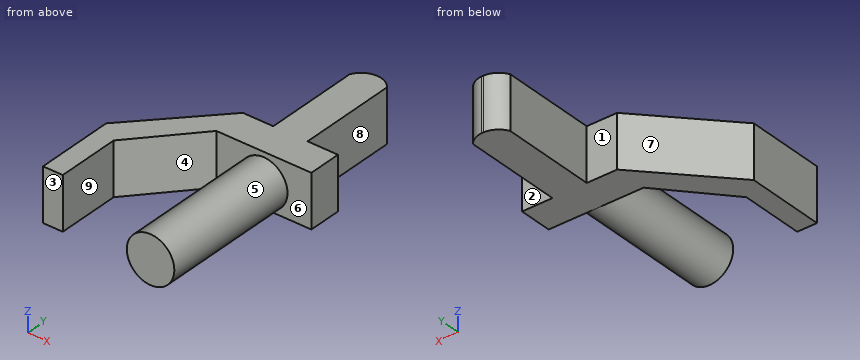
from build123d import *

# Parameters (mm, degrees)
BOSS_EXTRUDE1_DEPTH = 4
SKETCH_1_W          = 7.2
SKETCH_1_H          = 2.5
EXTRUDE_1_DEPTH     = 4
EXTRUDE_2_DEPTH     = 4
SKETCH_6_R          = 1.8
EXTRUDE_3_DEPTH     = 10.65


with BuildPart() as part:
    # Sketch1 → Boss-Extrude1 (new body)
    with BuildSketch(Plane.XY):
        with BuildLine():
            Line((-10.408670574, 3.576426588), (-7.808670574, 3.576426588))
            Line((-7.808670574, 3.576426588), (-7.808670574, 11.055036677))
            ThreePointArc((-7.808670574, 11.055036677), (-8.310608651, 11.480313821), (-8.944823261, 11.655168937))
            Line((-8.944823261, 11.655168937), (-9.103917888, 11.655168937))
            ThreePointArc((-9.103917888, 11.655168937), (-9.878044557, 11.396572098), (-10.408670574, 10.776426588))
            Line((-10.408670574, 10.776426588), (-10.408670574, 3.576426588))
        make_face()
    extrude(amount=BOSS_EXTRUDE1_DEPTH)

    # Эскиз1 → Бобышка-Вытянуть1 (add)
    with BuildSketch(Plane.XY.offset(4)):
        with Locations((-9.108670574, 2.329960492)):
            Rectangle(SKETCH_1_W, SKETCH_1_H)
    extrude(amount=-EXTRUDE_1_DEPTH)

    # Эскиз5 → Бобышка-Вытянуть2 (add)
    with BuildSketch(Plane.XY.offset(4)):
        Polygon((-12.708670574, 3.579960492), (-18.284126234, -2.357514059), (-18.284126234, -8.307514059), (-16.784126234, -8.307514059), (-16.784126234, -3.524992463), (-12.708670574, 1.079960492), align=None)
    extrude(amount=-EXTRUDE_2_DEPTH)

    # Эскиз6 → Бобышка-Вытянуть3 (add)
    with BuildSketch(Plane.XZ.offset(-1.079960492)):
        with Locations((-9.118354015, 1.82)):
            Circle(SKETCH_6_R)
    extrude(amount=EXTRUDE_3_DEPTH)


solid = part.part
CAD build for the part. Positions are in the model's coordinates, mm. Face numbers are marked on the shaded views. A direction names the side the tool comes from. Coordinates: 2 decimals unless noted, no trailing zeros. Loops run counter-clockwise (first coordinate to the right, second up) from the corner with the lowest first, then second, coordinate; pieces in that order, holes last. Notation, with made-up numbers: (49.5, 4.25) - (107.5, 4.25) arc R32 ccw to (107.5, 34.25) - close; hole circle Ø4 at (-20, 27). An arc over 180 degrees is marked (long way). Write item = value, one per line. Start each with the question number.
Q1. Drill centre lines: L1, parallel to X at y = -4.75, z = 3.15; L2, parallel to X at y = 3.75, z = 0.25; L3, parallel to X at y = -1.5, z = 0.55. Where is each one in solid material? Low to high.
Q2. Cut at B-B, the plane y = -5.75. List the corners of the cut face in (x, z).
Q3. Cut at D-D, the plane y = 9. List the corners of the cut face in (x, z).
Q4. Pull direction X, two halves, no side cores. Call the marked faces 6, 7, 8 and 9: pulls with the +X half, pulls with the -X half, needs draft (parallel to the pull), parting line crosses it, or undercut.
Q5. Cut at A-A, the plane z = 1.82. List the corners of the cut face in (x, y) (3 decimals).
Q6. Which spindle directions (+Z, -Z, +X, -X, +Y, -Y) get a long thin tool onto all of the face, cutting with end or side? Do the marked faces 1, 2, 3, 4 and 5. Say none if no direction does.
Q7. Flat gauge pins, fed straight in: pin 1 Ø1.2 at (x, z) = (-6.5, 1) entering from +Y; pin 2 Ø1.6 at (x, z) = (-17.5, 3) entering from -Y; pin 3 Ø1.2 at (y, z) = (8, 2) entering from -X. Where does each tip first touch, or does it go through?
Q8. Cut at C-C, the plane x = -17. List the corners of the cut face in (y, z).
Computed:
q1.L1 = -18.28 to -16.78, -10.33 to -7.91
q1.L2 = -10.41 to -7.81
q1.L3 = -17.48 to -14.99, -10.39 to -7.84
q2.outline = (-18.28, 0) - (-16.78, 0) - (-16.78, 4) - (-18.28, 4) - close; circle Ø3.6 at (-9.12, 1.82)
q3.outline = (-10.41, 0) - (-7.81, 0) - (-7.81, 4) - (-10.41, 4) - close
q4.face_6 = undercut
q4.face_7 = pulls with the -X half
q4.face_8 = pulls with the +X half
q4.face_9 = undercut
q5.outline = (-18.284, -8.308) - (-16.784, -8.308) - (-16.784, -3.525) - (-12.709, 1.08) - (-10.918, 1.08) - (-10.918, -9.57) - (-7.318, -9.57) - (-7.318, 1.08) - (-5.509, 1.08) - (-5.509, 3.58) - (-7.809, 3.58) - (-7.809, 11.055) arc R1.528 ccw to (-8.945, 11.655) - (-9.104, 11.655) arc R1.528 ccw to (-10.409, 10.776) - (-10.409, 3.58) - (-12.709, 3.58) - (-18.284, -2.358) - close
q6.face_1 = +Z, -Z, -X, +Y
q6.face_2 = +Z, -Z, +X, +Y
q6.face_3 = +Z, -Z, -X, -Y
q6.face_4 = +Z, -Z, -Y
q6.face_5 = -Y
q7.pin_1 = 3.58
q7.pin_2 = -8.31
q7.pin_3 = -10.41
q8.outline = (-8.31, 0) - (-0.99, 0) - (-0.99, 4) - (-8.31, 4) - close
